```python
from build123d import *

# Parameters (mm, degrees)
F0_W      = 33.02
F0_H      = 59.69
F1_DEPTH  = 5.08
F2_W      = 17.78
F2_H      = 5.08
F3_DEPTH  = 5.08
F4_R      = 0.889
F5_DEPTH  = 17.78
F6_R      = 2.53999
F7_W      = 27.94
F7_H      = 6.35
F8_DEPTH  = 6.35
F9_R      = 5.08
F10_W     = 25.4
F10_H     = 5.08
F11_DEPTH = 6.35


# Not quite as in the source:
# - a fillet or chamfer is up to 0.001 mm smaller than in the source, because OpenCascade refuses the exact size


with BuildPart() as f1:
    # F0 (on Top) → F1 (new body)
    with BuildSketch(Plane.XY):
        with Locations((16.51, 29.845)):
            Rectangle(F0_W, F0_H)
    extrude(amount=F1_DEPTH)

    # F2 (on face) → F3 (join)
    with BuildSketch(Plane(origin=(0, 59.69, 0), x_dir=(-1, 0, 0), z_dir=(0, 1, 0))):
        with Locations((-16.51, 2.54)):
            Rectangle(F2_W, F2_H)
    extrude(amount=F3_DEPTH)

    # F4 (on face) → F5 (cut)
    with BuildSketch(Plane(origin=(7.62, 0, 0), x_dir=(0, -1, 0), z_dir=(-1, 0, 0))):
        with Locations((-62.23, 2.54)):
            Circle(F4_R)
    extrude(amount=-F5_DEPTH, mode=Mode.SUBTRACT)

    # F6 (radius 2.54 in the source; OpenCascade refuses exactly that, so slightly less here)
    f6_edges = [f1.edges().sort_by_distance(p)[0] for p in [
        (16.51, 64.77, 0),
        (16.51, 64.77, 5.08),
    ]]
    fillet(f6_edges, radius=F6_R)

    # F7 (on face) → F8 (join)
    with BuildSketch(Plane.XY.offset(5.08)):
        with Locations((16.51, 5.715)):
            Rectangle(F7_W, F7_H)
    extrude(amount=F8_DEPTH)

    # F9
    f9_edges = [f1.edges().sort_by_distance(p)[0] for p in [
        (16.51, 2.54, 11.43),
    ]]
    fillet(f9_edges, radius=F9_R)

    # F10 (on face) → F11 (join)
    with BuildSketch(Plane.XZ):
        with Locations((16.51, 2.54)):
            Rectangle(F10_W, F10_H)
    extrude(amount=F11_DEPTH)


solid = f1.part
```
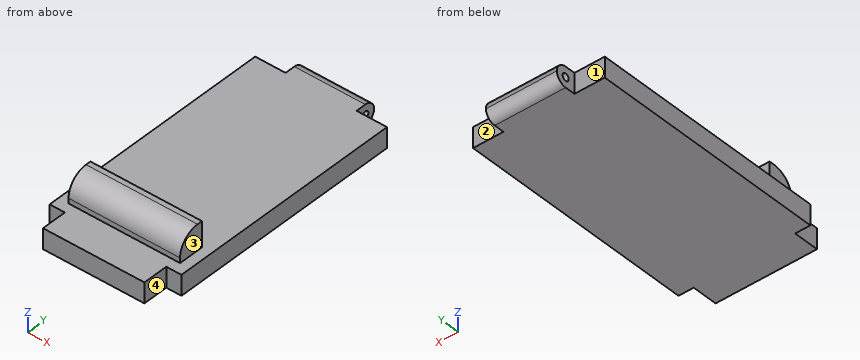
Input: part model. Units: mm. Frame: model coordinates. Face numbers are marked on the shaded views. A direction names the side the tool comes from. Round coordinates to 2 decimals unless told otherwise and drop trailing zeros. Loops run counter-clockwise (first coordinate to the right, second up) from the corner with the lowest first, then second, coordinate; pieces in that order, holes last.
1) Section query B-B on y = 15. Return the cut outline in (x, z).
Ans:
outline: (0, 0) - (33.02, 0) - (33.02, 5.08) - (0, 5.08) - close
2) Material intervals for line 1 (Z direction, x = 12.25, y = 62.23); line 2 (Z direction, x = 32, y = 41); line 3 (Y direction, x = 9.5, z = 1.75), sorted ascending.
Ans:
line 1: z = 0 to 1.65, 3.43 to 5.08
line 2: z = 0 to 5.08
line 3: y = -6.35 to 61.82, 62.64 to 64.64
3) Section query C-C on z = 7. Return the cut outline in (x, y).
Ans:
outline: (2.54, 2.58) - (30.48, 2.58) - (30.48, 8.89) - (2.54, 8.89) - close
4) Set-up query: the marked faces 1, 2, 3 and 4. Return all of +Z, -Z, +X, -X, +Y, -Y with unobstructed straight access to the full face (end or side cutting, diameter ignored); none if empty.
Ans:
face 1: +Z, -Z, -X, +Y
face 2: +Z, -Z, +X, +Y
face 3: +Z, +X, +Y, -Y
face 4: +Z, -Z, +X, -Y
5) Pin query (flat end, axial travel): pin 1 (1.5 mm diameter, centred on x = 8.5, y = 10, fed in from +Z); pin 2 (1.9 mm diameter, centred on x = 31.5, z = 3, fed in from -Y); pin 3 (1.5 mm diameter, centred on x = 3, z = 2.5, fed in from +Y). Return the tip coordinate at first contact, or that it passes through.
Ans:
pin 1: stops at z = 5.08
pin 2: stops at y = 0
pin 3: stops at y = 59.69
